Verification items for this drawing (mm, ordinates from the low corner). A direction names the side the tool comes from. Coordinates: 2 decimals unless noted, no trailing zeros. Write each loop counter-clockwise with the first axis right and the second up, starting at its lowest first coordinate (ties: lowest second). Pieces come first, ordered by that corner, then holes. Notation, with made-up numbers: (60.5, 28.25) -> (71.5, 28.25) arc R27 ccw to (71.5, 67.25) -> close; hole circle Ø10 at (-29, 21.5). An arc over 180 degrees is marked (long way). One line per question, with ' | ' between items.
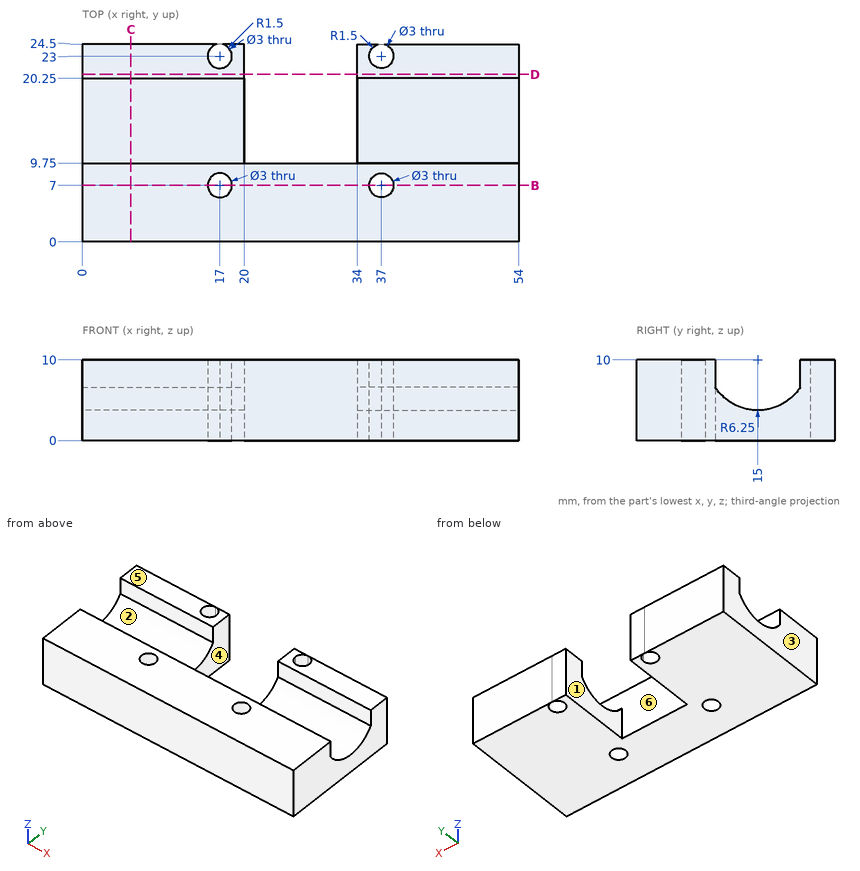
(1) Material ranges on line 1 (X direction, y = 23, z = 7); line 2 (Y direction, x = 8.5, z = 8.5); line 3 (Y direction, x = 31, z = 3), recorded low to high.
Answers below:
line 1: x = 0 to 15.5, 18.5 to 20, 34 to 35.5, 38.5 to 54 | line 2: y = 0 to 9.75, 20.25 to 24.5 | line 3: y = 0 to 9.75
(2) Draft check along X on the marked faces 1, 2 and 3. Enter one of: pulls with the +X half, pulls with the -X half, needs draft (parallel to the pull), parting line crosses it, or undercut.
Answers below:
face 1: undercut | face 2: needs draft | face 3: pulls with the -X half
(3) Cross-section at D-D (y = 20.75). Record the cut outline in (x, z), plus the area to 3 significant figures.
Answers below:
outline: (0, 0) -> (20, 0) -> (20, 10) -> (0, 10) -> close; (34, 0) -> (54, 0) -> (54, 10) -> (34, 10) -> close | area: 400 mm²
(4) Depth check by flat-ended pin: P1, Ø5, axis at x = 28, z = 2, coming from the +Y side; P2, Ø2.5, axis at x = 17, y = 7, coming from the +Z side; P3, Ø1, axis at x = 10, y = 14.5, coming from the +Z side. Enter the tip coordinate at first touch or a pass-through.
Answers below:
P1: stops at y = 9.75 | P2: passes through | P3: stops at z = 3.83
(5) Cross-section at B-B (y = 7). Record the cut outline in (x, z), plus the area to 3 significant figures.
Answers below:
outline: (0, 0) -> (15.5, 0) -> (15.5, 10) -> (0, 10) -> close; (18.5, 0) -> (35.5, 0) -> (35.5, 10) -> (18.5, 10) -> close; (38.5, 0) -> (54, 0) -> (54, 10) -> (38.5, 10) -> close | area: 480 mm²
(6) Cross-section at C-C (x = 6). Record the cut outline in (y, z), plus the area to 3 significant figures.
Answers below:
outline: (0, 0) -> (24.5, 0) -> (24.5, 10) -> (20.25, 10) -> (20.25, 6.61) arc R6.25 cw to (9.75, 6.61) -> (9.75, 10) -> (0, 10) -> close | area: 188 mm²
(7) Tool access check on the marked faces 4, 5 and 6. Record the directions out of +Z, -Z, +X, -X, +Y, -Y that give a thin tool (end or side, any length) a straight path to the whole face; none if there is none.
Answers below:
face 4: +Z, -Z, +Y | face 5: +Z, +X, -X, +Y, -Y | face 6: +Z
